Input: part model. Units: mm. Frame: model coordinates. Face numbers are marked on the shaded views. A direction names the side the tool comes from. Coordinates: 2 decimals unless noted, no trailing zeros. Loops run counter-clockwise (first coordinate to the right, second up) from the corner with the lowest first, then second, coordinate; pieces in that order, holes last. Notation, with made-up numbers: (-34, -31) -> (-25, -31) arc R7 cw to (-25, -22) -> close; hole circle Ø11 at (-18.5, 20.25). An arc over 180 degrees is marked (long way). Answer as a JSON object with one key per item and string values.
from build123d import *

# Parameters (mm, degrees)
F2_DEPTH        = 10
F2_COPIES_COUNT = 12
F4_R            = 7
F5_DEPTH        = 20.001


# Not quite as in the source:
# - a feature of the source that left no trace in its solid (it failed there, or was rolled back) is left out
# - a pattern or mirror of a feature is missing from the dataset's text; its kind, count and spacing are read off the source's solid


with BuildPart() as f2:
    # F1 (on Front) → F2 (new body, symmetric)
    with BuildSketch(Plane.XZ):
        with BuildLine():
            ThreePointArc((-2.6105238444, 19.8288972275), (-13.186916302, -15.0367961496), (20, 0))
            ThreePointArc((20, 0), (15.0367961496, 13.186916302), (2.6105238444, 19.8288972275))
            ThreePointArc((2.6105238444, 19.8288972275), (0, 20), (-2.6105238444, 19.8288972275))
        make_face()
        with BuildLine():
            ThreePointArc((-2.6105238444, 19.8288972275), (0, 20), (2.6105238444, 19.8288972275))
            Line((2.6105238444, 19.8288972275), (3.1326286133, 23.794676673))
            ThreePointArc((3.1326286133, 23.794676673), (2.0019466325, 26.1165955987), (0, 27.7481466766))
            ThreePointArc((0, 27.7481466766), (-2.0019466325, 26.1165955987), (-3.1326286133, 23.794676673))
            Line((-3.1326286133, 23.794676673), (-2.6105238444, 19.8288972275))
        make_face()
    extrude(amount=F2_DEPTH, both=True)

    # F2_copies: F2 ×12 about axis
    f2_copies_axis = Axis((0, 0, 0), (0, 1, 0))


with BuildPart() as f2_1:
    add(f2.part)
    for i in range(1, F2_COPIES_COUNT):
        add(f2.part.rotate(f2_copies_axis, i * 360 / F2_COPIES_COUNT))

    # F4 (on face) → F5 (cut, through all)
    with BuildSketch(Plane.XZ.offset(10)):
        Circle(F4_R)
    extrude(amount=-F5_DEPTH, mode=Mode.SUBTRACT)


solid = f2_1.part
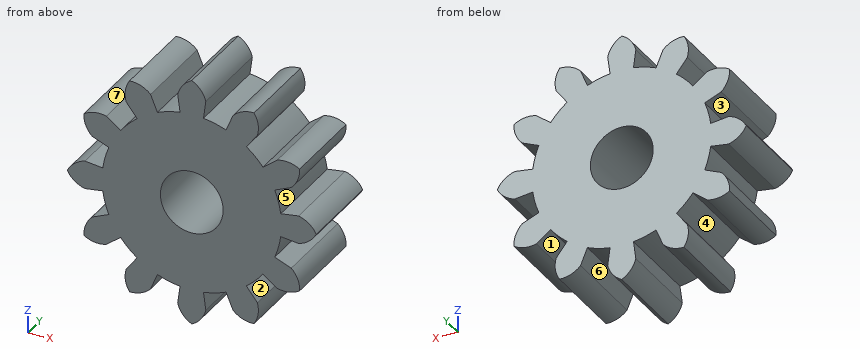
1. Mould query, pull axis Z, two halves, no side actions, for the marked faces 5, 6 and 7. Classes: pulls with the +Z half, pulls with the -Z half, needs draft (parallel to the pull), parting line crosses it, or undercut.
Reply:
{"face 5": "undercut", "face 6": "pulls with the -Z half", "face 7": "pulls with the +Z half"}
2. Section query C-C (x = -5). Return loops of the section in (y, z).
Reply:
{"outline": "(-10, -19.36) -> (10, -19.36) -> (10, -4.9) -> (-10, -4.9) -> close; (-10, 4.9) -> (10, 4.9) -> (10, 19.36) -> (-10, 19.36) -> close"}
3. Pin query (flat end, axial travel): P1, Ø1, axis at x = -13, y = -4, coming from the -Z side; P2, Ø2, axis at x = -1.5, y = -4.5, coming from the +Z side; P3, Ø10, axis at x = -6.5, y = -3, coming from the -Z side; P4, Ø8.5, axis at x = 0, z = 0, coming from the +Y side. Return the tip coordinate at first contact, or that it passes through.
Reply:
{"P1": "stops at z = -24.04", "P2": "stops at z = 27.47", "P3": "stops at z = -26.67", "P4": "passes through"}
4. Access query for the marked faces 1, 2, 3 and 4. Directions: +Z, -Z, +X, -X, +Y, -Y. A direction counts if a zero-diameter tool reaches every point of the face in a straight line with its end or side. Return the directions, or none.
Reply:
{"face 1": "-Z, +Y, -Y", "face 2": "+X, +Y, -Y", "face 3": "-X, +Y, -Y", "face 4": "+Y, -Y"}
5. Section query A-A (x = 13). Return loops of the section in (y, z), plus the area to 3 significant figures.
Reply:
{"outline": "(-10, -24.02) -> (10, -24.02) -> (10, -16.94) -> (-10, -16.94) -> close; (-10, -15.2) -> (10, -15.2) -> (10, 15.2) -> (-10, 15.2) -> close; (-10, 16.94) -> (10, 16.94) -> (10, 24.02) -> (-10, 24.02) -> close", "area": "891 mm2"}
6. Line query: line 1 along X through (y, z) = (-1, 20); line 2 along Z through (x, y) = (-13, -5.5); line 3 along Z through (x, y) = (-1, -5.75). Output: solid intervals per line, ascending.
Reply:
{"line 1": "x = -14.81 to -8.28, -2.63 to 2.63, 8.28 to 14.81", "line 2": "z = -24.02 to -16.94, -15.2 to 15.2, 16.94 to 24.02", "line 3": "z = -27.11 to -6.93, 6.93 to 27.11"}
7. Section query D-D (x = -21.5). Return loops of the section in (y, z).
Reply:
{"outline": "(-10, -14.81) -> (10, -14.81) -> (10, -8.91) -> (-10, -8.91) -> close; (-10, -2.83) -> (10, -2.83) -> (10, 2.83) -> (-10, 2.83) -> close; (-10, 8.91) -> (10, 8.91) -> (10, 14.81) -> (-10, 14.81) -> close"}
8. Section query B-B (z = 1). Return loops of the section in (x, y), plus the area to 3 significant figures.
Reply:
{"outline": "(-27.11, -10) -> (-6.93, -10) -> (-6.93, 10) -> (-27.11, 10) -> close; (6.93, -10) -> (27.11, -10) -> (27.11, 10) -> (6.93, 10) -> close", "area": "807 mm2"}
